Here's how the part is built. I have some questions about the finished solid (model axes, mm). Face numbers are marked on the shaded views. A direction names the side the tool comes from. Give positions to 0.01 mm unless a question says otherwise; leave off trailing zeros. Loops run counter-clockwise (first coordinate to the right, second up) from the corner with the lowest first, then second, coordinate; pieces in that order, holes last.
Q1. Suppose I cut it at C-C (x = 8.25). List the corners of the cut face in (y, z) for me, and give its area (3 significant figures).
Q2. Suppose I cut it at D-D (y = 25). List the corners of the cut face in (x, z) for me, and give its area (3 significant figures).
Q3. I need wall thicknesses on probe 1 along Z at (x, y) = (0, 8.55); probe 2 along Y at (x, z) = (-11.5, 41); probe 3 along Z at (x, y) = (6.25, 31). Which ranges of each line are inside material? Lowest first, please.
Q4. Suppose I cut it at A-A (z = 22). List the corners of the cut face in (x, y) for me.
Q5. Thinking about a two-plate mould opening in X: for the marked faces 3, 4, 5 and 6, which applies, pulls with the +X half, pulls with the -X half, needs draft (parallel to the pull), parting line crosses it, or undercut?
Q6. Suppose I cut it at B-B (x = 0). List the corners of the cut face in (y, z) for me.
Q7. I'm going to push flat-ended pins straight in: P1, Ø4.5, axis at x = 8.12, y = 28.55, coming from the +Z side; P2, Ø8, axis at x = 0, z = 22, coming from the +Y side; P3, Ø2, axis at x = -8.12, y = 15.45, coming from the +Z side. Where does each tip first touch, or does it pass through?
Q8. For the marked faces 1 and 2, which set-ups out of +Z, -Z, +X, -X, +Y, -Y let a thin tool reach every point of the face, with its end or its side?
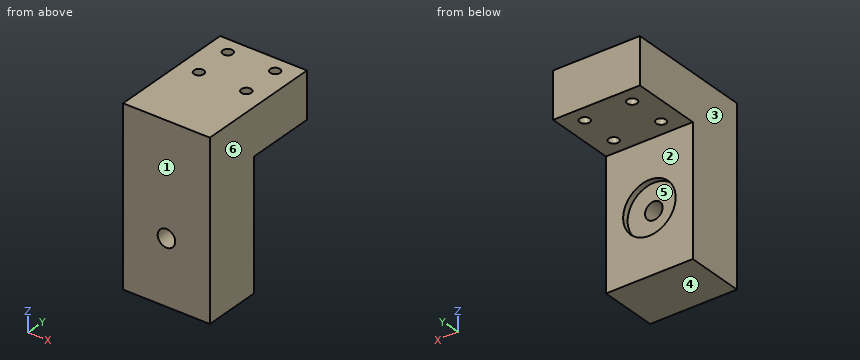
```python
from build123d import *

# Parameters (mm, degrees)
SKETCH1_W           = 29.78
SKETCH1_H           = 20
BOSS_EXTRUDE2_DEPTH = 44
SKETCH4_W           = 29.78
SKETCH4_H           = 44
BOSS_EXTRUDE3_DEPTH = 15.87
SKETCH5_R           = 9
CUT_EXTRUDE1_DEPTH  = 2
SKETCH7_R           = 3.0125
CUT_EXTRUDE2_DEPTH  = 67.948704244
SKETCH8_R           = 1.7
CUT_EXTRUDE3_DEPTH  = 58.564851255


with BuildPart() as part:
    # Sketch1 → Boss-Extrude2 (new body)
    with BuildSketch(Plane.XY):
        Rectangle(SKETCH1_W, SKETCH1_H)
    extrude(amount=BOSS_EXTRUDE2_DEPTH)

    # Sketch4 → Boss-Extrude3 (add)
    with BuildSketch(Plane.XY.offset(44)):
        with Locations((0, 12)):
            Rectangle(SKETCH4_W, SKETCH4_H)
    extrude(amount=BOSS_EXTRUDE3_DEPTH)

    # Sketch5 → Cut-Extrude1 (cut)
    with BuildSketch(Plane(origin=(0, 10, 0), x_dir=(1, 0, 0), z_dir=(0, 1, 0))):
        with Locations(Location((0, -22, 0), (0, 0, 180))):
            Circle(SKETCH5_R)
    extrude(amount=-CUT_EXTRUDE1_DEPTH, mode=Mode.SUBTRACT)

    # Sketch7 → Cut-Extrude2 (cut, through all)
    with BuildSketch(Plane(origin=(0, 8, 0), x_dir=(1, 0, 0), z_dir=(0, 1, 0))):
        with Locations(Location((0, -22, 0), (0, 0, 180))):
            Circle(SKETCH7_R)
    extrude(amount=-CUT_EXTRUDE2_DEPTH, mode=Mode.SUBTRACT)

    # Sketch8 → Cut-Extrude3 (cut, through all)
    with BuildSketch(Plane(origin=(0, 0, 44), x_dir=(-1, 0, 0), z_dir=(0, 0, -1))):
        with Locations((-8.123713821, 28.54698226)):
            Circle(SKETCH8_R)
        with Locations((8.123713821, 28.54698226)):
            Circle(SKETCH8_R)
        with Locations((-8.123713821, 15.45301774)):
            Circle(SKETCH8_R)
        with Locations((8.123713821, 15.45301774)):
            Circle(SKETCH8_R)
    extrude(amount=-CUT_EXTRUDE3_DEPTH, mode=Mode.SUBTRACT)


solid = part.part
```
Solutions:
1. outline: (-10, 0) - (10, 0) - (10, 18.4) - (8, 18.4) - (8, 25.6) - (10, 25.6) - (10, 44) - (13.76, 44) - (13.76, 59.87) - (-10, 59.87) - close; (17.15, 44) - (26.85, 44) - (26.85, 59.87) - (17.15, 59.87) - close; (30.24, 44) - (34, 44) - (34, 59.87) - (30.24, 59.87) - close
1. area: 1,460 mm2
2. outline: (-14.89, 44) - (14.89, 44) - (14.89, 59.87) - (-14.89, 59.87) - close
2. area: 473 mm2
3. probe 1: z = 0 to 13, 31 to 59.87
3. probe 2: y = -10 to 10
3. probe 3: z = 44 to 59.87
4. outline: (-14.89, -10) - (-3.01, -10) - (-3.01, 8) - (-9, 8) - (-9, 10) - (-14.89, 10) - close; (3.01, -10) - (14.89, -10) - (14.89, 10) - (9, 10) - (9, 8) - (3.01, 8) - close
5. face 3: pulls with the -X half
5. face 4: needs draft
5. face 5: undercut
5. face 6: pulls with the +X half
6. outline: (-10, 0) - (10, 0) - (10, 13) - (8, 13) - (8, 18.99) - (-10, 18.99) - close; (-10, 25.01) - (8, 25.01) - (8, 31) - (10, 31) - (10, 44) - (34, 44) - (34, 59.87) - (-10, 59.87) - close
7. P1: stops at z = 59.87
7. P2: stops at y = 8
7. P3: passes through
8. face 1: +Z, -Z, +X, -X, -Y
8. face 2: -Z, +X, -X, +Y
